Verification items for the finished model (mm, model axes). Face numbers are marked on the shaded views. A direction names the side the tool comes from. Give positions to 0.01 mm unless a question says otherwise; leave off trailing zeros. Write each loop counter-clockwise with the first axis right and the second up, starting at its lowest first coordinate (ties: lowest second). Pieces come first, ordered by that corner, then holes. Notation, with made-up numbers: M 66,31 L 120,31 A31 ccw 120,61 Z; hole C -29,66 d1. An arc over 180 degrees is marked long. Write item = value, one per line.
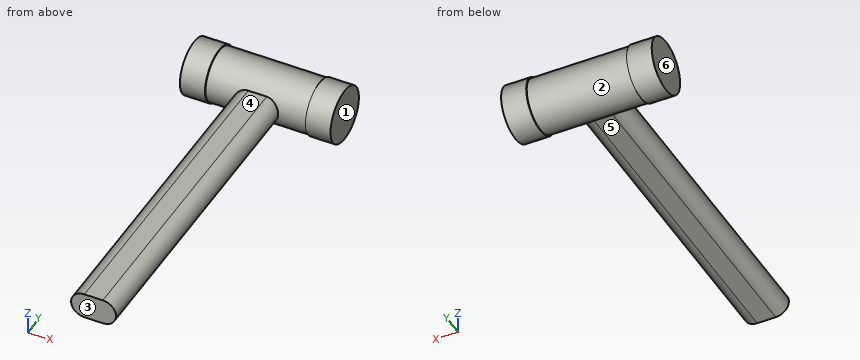
from build123d import *

# Parameters (mm, degrees)
SKIZZE1_W                       = 76
SKIZZE1_H                       = 20.25
AUFSATZ_LINEAR_AUSTRAGEN1_DEPTH = 260


with BuildPart() as part:
    # Skizze1 → Rotation1 (revolve)
    with BuildSketch(Plane.XY, mode=Mode.PRIVATE) as rotation1_sk:
        with Locations((0, 10.125)):
            Rectangle(SKIZZE1_W, SKIZZE1_H)
        Polygon((-57, 21), (-57, 0), (-38, 0), (-38, 20.25), (-38, 21), align=None)
        Polygon((38, 20.25), (38, 0), (57, 0), (57, 21), (38, 21), align=None)
    revolve(rotation1_sk.sketch.rotate(Axis((-67.247528095, 0, 0), (1, 0, 0)), 90), axis=Axis((-67.247528095, 0, 0), (1, 0, 0)))

    # Skizze2 → Aufsatz-Linear austragen1 (add)
    with BuildSketch(Plane(origin=(0, 0, 0), x_dir=(1, 0, 0), z_dir=(0, 1, 0))):
        with BuildLine():
            Line((-7, 10), (7, 10))
            ThreePointArc((7, 10), (17, 0), (7, -10))
            Line((7, -10), (-7, -10))
            ThreePointArc((-7, -10), (-17, 0), (-7, 10))
        make_face()
    extrude(amount=-AUFSATZ_LINEAR_AUSTRAGEN1_DEPTH)


solid = part.part
1) Tool access check on the marked faces 4, 5 and 6. Record the directions out of +Z, -Z, +X, -X, +Y, -Y that give a thin tool (end or side, any length) a straight path to the whole face; none if there is none.
From the geometry:
face_4 = +Z, +X, -X, -Y
face_5 = -Z, +X, -X, -Y
face_6 = +Z, -Z, -X, +Y, -Y
2) Cross-section at B-B on y = 0. Record the boundary of the cut face in (x, z), plus the area to 3 significant figures.
From the geometry:
outline = M -57,-21 L -38,-21 L -38,-20.25 L 38,-20.25 L 38,-21 L 57,-21 L 57,21 L 38,21 L 38,20.25 L -38,20.25 L -38,21 L -57,21 Z
area = 4,670 mm^2
3) Cross-section at A-A on z = 0. Record the boundary of the cut face in (x, y), plus the area to 3 significant figures.
From the geometry:
outline = M -57,-21 L -38,-21 L -38,-20.25 L -17,-20.25 L -17,-260 L 17,-260 L 17,-20.25 L 38,-20.25 L 38,-21 L 57,-21 L 57,21 L 38,21 L 38,20.25 L -38,20.25 L -38,21 L -57,21 Z
area = 12,800 mm^2
4) Material ranges on probe 1 along Z at (x, y) = (-3, -18); probe 2 along X at (y, z) = (-85, -3); probe 3 along Y at (x, z) = (-33.5, 16.5), recorded low to high. Write a range as from..to.
From the geometry:
probe_1 = -10..10
probe_2 = -16.54..16.54
probe_3 = -11.74..11.74
5) Cross-section at C-C on x = 24. Record the boundary of the cut face in (y, z).
From the geometry:
outline = C 0,0 d40.5
6) Cross-section at D-D on y = -89.5. Record the boundary of the cut face in (x, z), plus the area to 3 significant figures.
From the geometry:
outline = M -7,-10 L 7,-10 A10 ccw 7,10 L -7,10 A10 ccw Z
area = 594 mm^2
7) Draft check along X on the marked faces 1, 2 and 3. Enter one of: +X half, -X half, draft (parallel to the pull), parting line (faces both ways), or undercut.
From the geometry:
face_1 = +X half
face_2 = undercut
face_3 = draft
8) Depth check by flat-ended pin: P1, Ø12, axis at x = 4.5, y = -213.5, coming from the +Z side; P2, Ø10, axis at x = 13.5, y = -219.5, coming from the +Z side; P3, Ø5, axis at x = -16.5, z = 1, coming from the +Y side. Enter the tip coordinate at first touch or a pass-through.
From the geometry:
P1 = 10
P2 = 9.89
P3 = 20.25
